Build history of the part. All positions in model axes, mm. Face numbers are marked on the shaded views. A direction names the side the tool comes from. Coordinates: 2 decimals unless noted, no trailing zeros. Loops run counter-clockwise (first coordinate to the right, second up) from the corner with the lowest first, then second, coordinate; pieces in that order, holes last.
Item 1: Drill centre lines: line 1 along X through (y, z) = (-6, 12); line 2 along X through (y, z) = (0, 6.5); line 3 along X through (y, z) = (3.25, 4.5). Where is each one in solid material? Low to high.
Item 2: 3-axis set-ups, long thin cutter, end or side, ignore diameter. For the marked faces 5, 6 and 7: which of +Z, -Z, +X, -X, +Y, -Y reach the whole face in a straight line?
Item 3: Cut at A-A (y = 0). List the corners of the cut face in (x, z), and give its area (3 significant figures).
Item 4: Cut at C-C (x = 4.5). List the corners of the cut face in (y, z), and give its area (3 significant figures).
Item 5: Cut at D-D (z = 7.25). List the corners of the cut face in (x, y), and give its area (3 significant figures).
Item 6: Flat gauge pins, fed straight in: pin 1 (3 mm diameter, centred on x = -1.5, z = 10.5, fed in from +Y); pin 2 (5 mm diameter, centred on x = -13.5, y = 0.5, fed in from +Z); pin 3 (6.5 mm diameter, centred on x = -0.5, y = -2.5, fed in from -Z). Where does each tip first touch, or does it go through?
Item 7: Mould opens along Y. For the marked faces 1, 2, 3 and 4 say: released by +Y, released by -Y, zero draft, split by the parting line, or undercut.
Item 8: Cut at B-B (z = 12). List the corners of the cut face in (x, y).
from build123d import *

# Parameters (mm, degrees)
SKETCH1_W           = 38
SKETCH1_H           = 13
BOSS_EXTRUDE1_DEPTH = 8
SKETCH2_W           = 19
SKETCH2_H           = 14
CUT_EXTRUDE1_DEPTH  = 9
SKETCH3_R           = 2
CUT_EXTRUDE2_DEPTH  = 9
SKETCH4_W           = 19
SKETCH4_H           = 6
BOSS_EXTRUDE2_DEPTH = 8
SKETCH5_R           = 1.75
CUT_EXTRUDE3_DEPTH  = 7
CUT_EXTRUDE4_DEPTH  = 4
SKETCH7_W           = 16
SKETCH7_H           = 10
CUT_EXTRUDE5_DEPTH  = 4
CHAMFER1_SIZE       = 2
SKETCH8_W           = 19
SKETCH8_H           = 2
CUT_EXTRUDE6_DEPTH  = 7


with BuildPart() as part:
    # Sketch1 → Boss-Extrude1 (new body)
    with BuildSketch(Plane.XY):
        Rectangle(SKETCH1_W, SKETCH1_H)
    extrude(amount=BOSS_EXTRUDE1_DEPTH)

    # Sketch2 → Cut-Extrude1 (cut, through all)
    with BuildSketch(Plane.XY.offset(8)):
        with Locations((0, 6.5)):
            Rectangle(SKETCH2_W, SKETCH2_H)
    extrude(amount=-CUT_EXTRUDE1_DEPTH, mode=Mode.SUBTRACT)

    # Sketch3 → Cut-Extrude2 (cut, through all)
    with BuildSketch(Plane.XY.offset(8)):
        with Locations((-13, 0)):
            Circle(SKETCH3_R)
        with Locations((13, 0)):
            Circle(SKETCH3_R)
    extrude(amount=-CUT_EXTRUDE2_DEPTH, mode=Mode.SUBTRACT)

    # Sketch4 → Boss-Extrude2 (add)
    with BuildSketch(Plane.XY.offset(8)):
        with Locations((0, -3.5)):
            Rectangle(SKETCH4_W, SKETCH4_H)
    extrude(amount=BOSS_EXTRUDE2_DEPTH)

    # Sketch5 → Cut-Extrude3 (cut, through all)
    with BuildSketch(Plane(origin=(0, -0.5, 0), x_dir=(1, 0, 0), z_dir=(0, 1, 0))):
        with Locations((-4.5, -12)):
            Circle(SKETCH5_R)
        with Locations((4.5, -12)):
            Circle(SKETCH5_R)
    extrude(amount=-CUT_EXTRUDE3_DEPTH, mode=Mode.SUBTRACT)

    # Sketch6 → Cut-Extrude4 (cut)
    with BuildSketch(Plane.XY.offset(8)):
        Polygon((-13, 3.464101615), (-16, 1.732050808), (-16, -1.732050808), (-13, -3.464101615), (-10, -1.732050808), (-10, 1.732050808), align=None)
        Polygon((13, -3.464101615), (16, -1.732050808), (16, 1.732050808), (13, 3.464101615), (10, 1.732050808), (10, -1.732050808), align=None)
    extrude(amount=-CUT_EXTRUDE4_DEPTH, mode=Mode.SUBTRACT)

    # Sketch7 → Cut-Extrude5 (cut)
    with BuildSketch(Plane(origin=(0, -0.5, 0), x_dir=(1, 0, 0), z_dir=(0, 1, 0))):
        with Locations((0, -11)):
            Rectangle(SKETCH7_W, SKETCH7_H)
    extrude(amount=-CUT_EXTRUDE5_DEPTH, mode=Mode.SUBTRACT)

    # Chamfer1
    chamfer1_edges = [part.edges().sort_by_distance(p)[0] for p in [
        (-8.75, -0.5, 16),
        (8.75, -0.5, 16),
        (19, -6.5, 4),
        (-19, -6.5, 4),
        (-19, 6.5, 4),
        (19, 6.5, 4),
    ]]
    chamfer(chamfer1_edges, length=CHAMFER1_SIZE)

    # Sketch8 → Cut-Extrude6 (cut, through all)
    with BuildSketch(Plane(origin=(0, -0.5, 0), x_dir=(1, 0, 0), z_dir=(0, 1, 0))):
        with Locations((0, -1)):
            Rectangle(SKETCH8_W, SKETCH8_H)
    extrude(amount=-CUT_EXTRUDE6_DEPTH, mode=Mode.SUBTRACT)


solid = part.part
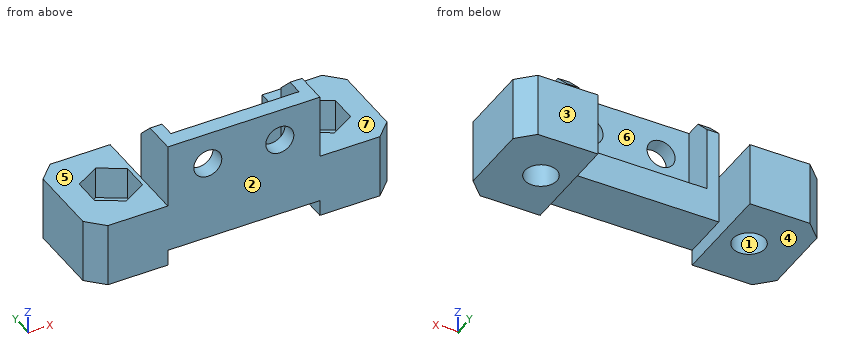
Filled sheet:
1. line 1: x = -9.5 to -6.25, -2.75 to 2.75, 6.25 to 9.5
1. line 2: x = -19 to -16, -10 to -9.5, 9.5 to 10, 16 to 19
1. line 3: x = -19 to -13.37, -12.63 to -9.5, 9.5 to 12.63, 13.37 to 19
2. face 5: +Z, -X, +Y, -Y
2. face 6: +Z, +Y
2. face 7: +Z, +X, +Y, -Y
3. outline: (-19, 0) - (-15, 0) - (-15, 4) - (-16, 4) - (-16, 8) - (-19, 8) - close; (-11, 0) - (-9.5, 0) - (-9.5, 8) - (-10, 8) - (-10, 4) - (-11, 4) - close; (9.5, 0) - (11, 0) - (11, 4) - (10, 4) - (10, 8) - (9.5, 8) - close; (15, 0) - (19, 0) - (19, 8) - (16, 8) - (16, 4) - (15, 4) - close
3. area: 72.0 mm2
4. outline: (-6.5, 2) - (-0.5, 2) - (-0.5, 6) - (-4.5, 6) - (-4.5, 10.25) - (-6.5, 10.25) - close; (-6.5, 13.75) - (-4.5, 13.75) - (-4.5, 16) - (-6.5, 16) - close
4. area: 37.0 mm2
5. outline: (-19, -4.5) - (-17, -6.5) - (17, -6.5) - (19, -4.5) - (19, 4.5) - (17, 6.5) - (9.5, 6.5) - (9.5, -0.5) - (8, -0.5) - (8, -4.5) - (-8, -4.5) - (-8, -0.5) - (-9.5, -0.5) - (-9.5, 6.5) - (-17, 6.5) - (-19, 4.5) - close; hole (-16, -1.73) - (-13, -3.46) - (-10, -1.73) - (-10, 1.73) - (-13, 3.46) - (-16, 1.73) - close; hole (10, -1.73) - (13, -3.46) - (16, -1.73) - (16, 1.73) - (13, 3.46) - (10, 1.73) - close
5. area: 227 mm2
6. pin 1: stops at y = -4.5
6. pin 2: stops at z = 8
6. pin 3: stops at z = 2
7. face 1: undercut
7. face 2: released by -Y
7. face 3: released by +Y
7. face 4: zero draft
8. outline: (-9.5, -6.5) - (-6.25, -6.5) - (-6.25, -4.5) - (-8, -4.5) - (-8, -0.5) - (-9.5, -0.5) - close; (-2.75, -6.5) - (2.75, -6.5) - (2.75, -4.5) - (-2.75, -4.5) - close; (6.25, -6.5) - (9.5, -6.5) - (9.5, -0.5) - (8, -0.5) - (8, -4.5) - (6.25, -4.5) - close
